Source: CAD feature listing. Evaluate the final solid. Frame: model axes, mm. Face numbers are marked on the shaded views. A direction names the side the tool comes from. Give positions to 0.01 mm unless a question says otherwise; leave off trailing zeros. Write each loop counter-clockwise with the first axis right and the second up, starting at its lowest first coordinate (ties: lowest second). Pieces come first, ordered by that corner, then holes. Notation, with made-up numbers: (58, 19) -> (88, 19) arc R9 cw to (88, 33) -> close; hole circle Ø6 at (55.25, 9). An arc over 180 degrees is marked (long way). Answer as a JSON object with one key per item and string values. Group by question number.
Item 1: Section query B-B on y = 6. Return the cut outline in (x, z) (3 decimals), plus the area to 3 significant figures.
Item 2: Access query for the marked faces 1, 2 and 3. Directions: +Z, -Z, +X, -X, +Y, -Y. A direction counts if a zero-diameter tool reaches every point of the face in a straight line with its end or side. Return the directions, or none.
Item 3: Ray query, probe 1 along Y at (x, z) = (0, 1.2) (3 decimals); probe 2 along Y at (x, z) = (0, 2.05); probe 3 along Z at (x, y) = (-4.75, -6.5). Return the intervals inside material, ascending. Write a range as from..to.
Item 4: Pull-direction query (X, two-part tool) for the marked faces 4, 5 and 6; classes: pulls with the +X half, pulls with the -X half, needs draft (parallel to the pull), parting line crosses it, or undercut.
Item 5: Section query C-C on x = 6.5. Return the cut outline in (y, z) (3 decimals), plus the area to 3 significant figures.
Item 6: Section query A-A on x = 0. Give the number of separate pieces and of enclosed holes in the cut face, plus the area to 4 significant figures.
Item 7: First-contact query: pin 1 Ø4 at (x, y) = (0, 0) entering from +Z; pin 2 Ø2 at (x, z) = (4, 2) entering from +Y; pin 3 Ø3 at (x, y) = (0.5, 0.5) entering from -Z. Flat tips, straight axial feed; report the tip coordinate or a pass-through.
Item 8: Section query D-D on z = -0.5. Return the cut outline in (x, y), plus the area to 3 significant figures.
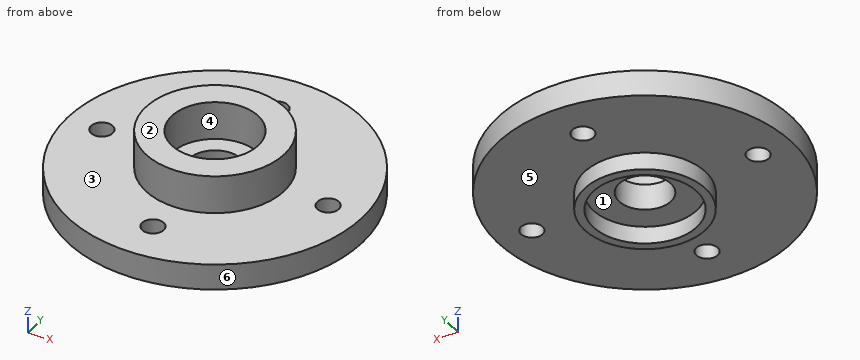
from build123d import *

# Parameters (mm, degrees)
SKETCH1_R           = 8.5
BOSS_EXTRUDE1_DEPTH = 1.5
SKETCH2_R           = 4
SKETCH2_R_2         = 2.5
BOSS_EXTRUDE2_DEPTH = 3.7
SKETCH3_R           = 1.5
CUT_EXTRUDE1_DEPTH  = 2
SKETCH4_R           = 0.625
CUT_EXTRUDE2_DEPTH  = 2
CIRPATTERN1_COUNT   = 2
SKETCH5_R           = 0.625
CUT_EXTRUDE3_DEPTH  = 1.5
SKETCH6_R           = 3.5
SKETCH6_R_2         = 3
BOSS_EXTRUDE3_DEPTH = 1


with BuildPart() as part:
    # Sketch1 → Boss-Extrude1 (new body)
    with BuildSketch(Plane.XY):
        Circle(SKETCH1_R)
    extrude(amount=BOSS_EXTRUDE1_DEPTH)

    # Sketch2 → Boss-Extrude2 (add)
    with BuildSketch(Plane.XY):
        Circle(SKETCH2_R)
        Circle(SKETCH2_R_2, mode=Mode.SUBTRACT)
    extrude(amount=BOSS_EXTRUDE2_DEPTH)

    # Sketch3 → Cut-Extrude1 (cut)
    with BuildSketch(Plane.XY):
        Circle(SKETCH3_R)
    extrude(amount=CUT_EXTRUDE1_DEPTH, mode=Mode.SUBTRACT)

    # Sketch4 → Cut-Extrude2 (cut)
    with BuildSketch(Plane.XY):
        with Locations((6.5, 0)):
            Circle(SKETCH4_R)
    cut_extrude2 = extrude(amount=CUT_EXTRUDE2_DEPTH, mode=Mode.SUBTRACT)

    # CirPattern1: Cut-Extrude2 ×2 about axis
    cirpattern1_axis = Axis((0, 0, 0), (0, 0, 1))
    for i in range(1, CIRPATTERN1_COUNT):
        add(cut_extrude2.rotate(cirpattern1_axis, i * 360 / CIRPATTERN1_COUNT), mode=Mode.SUBTRACT)

    # Sketch5 → Cut-Extrude3 (cut)
    with BuildSketch(Plane(origin=(0, 0, 0), x_dir=(-1, 0, 0), z_dir=(0, 0, -1))):
        with Locations((0, 6)):
            Circle(SKETCH5_R)
        with Locations((0, -6)):
            Circle(SKETCH5_R)
    extrude(amount=-CUT_EXTRUDE3_DEPTH, mode=Mode.SUBTRACT)

    # Sketch6 → Boss-Extrude3 (add)
    with BuildSketch(Plane(origin=(0, 0, 0), x_dir=(-1, 0, 0), z_dir=(0, 0, -1))):
        with Locations(Location((0, 0, 0), (0, 0, 180))):
            Circle(SKETCH6_R)
        Circle(SKETCH6_R_2, mode=Mode.SUBTRACT)
    extrude(amount=BOSS_EXTRUDE3_DEPTH)


solid = part.part
Worked answers:
{
 "1": {"outline": "(-6.021, 0) -> (-0.625, 0) -> (-0.625, 1.5) -> (-6.021, 1.5) -> close; (0.625, 0) -> (6.021, 0) -> (6.021, 1.5) -> (0.625, 1.5) -> close", "area": "16.2 mm^2"},
 "2": {"face 1": "-Z", "face 2": "+Z, +X, -X, +Y, -Y", "face 3": "+Z"},
 "3": {"probe 1": "-8.5..-6.625, -5.375..-1.5, 1.5..5.375, 6.625..8.5", "probe 2": "-4..-2.5, 2.5..4", "probe 3": "0..1.5"},
 "4": {"face 4": "undercut", "face 5": "needs draft", "face 6": "parting line crosses it"},
 "5": {"outline": "(-5.477, 0) -> (-0.625, 0) -> (-0.625, 1.5) -> (-5.477, 1.5) -> close; (0.625, 0) -> (5.477, 0) -> (5.477, 1.5) -> (0.625, 1.5) -> close", "area": "14.6 mm^2"},
 "6": {"separate pieces": "4", "enclosed holes": "0", "area": "24.85 mm^2"},
 "7": {"pin 1": "z = 1.5", "pin 2": "y = 7.9", "pin 3": "z = 0"},
 "8": {"outline": "circle Ø7 at (0, 0); hole circle Ø6 at (0, 0)", "area": "10.2 mm^2"}
}
